Part model, mm, in its own coordinate system. Face numbers are marked on the shaded views. A direction names the side the tool comes from. Round coordinates to 2 decimals unless told otherwise and drop trailing zeros. Loops run counter-clockwise (first coordinate to the right, second up) from the corner with the lowest first, then second, coordinate; pieces in that order, holes last. Notation, with made-up numbers: M -2,32.5 L 37,32.5 A37 ccw 37,68.5 Z; hole C 55,28 d8. An arc over 180 degrees is marked long. Write each question's results on one line, items separated by ' | '.
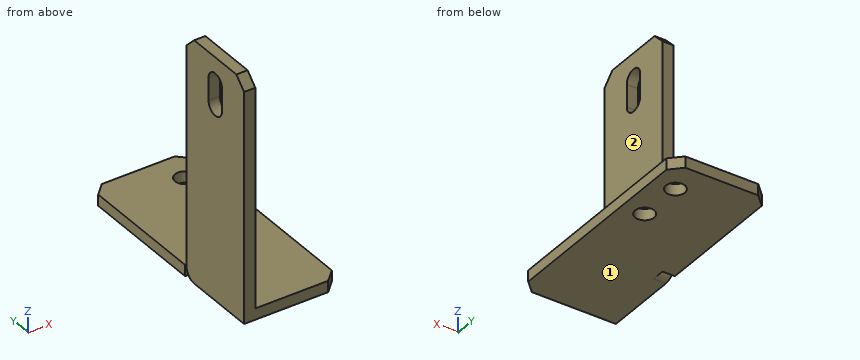
from build123d import *

# Parameters (mm, degrees)
SKETCH1_R           = 1.7
BOSS_EXTRUDE1_DEPTH = 2
SKETCH2_W           = 2
SKETCH2_H           = 15
BOSS_EXTRUDE2_DEPTH = 41
CUT_EXTRUDE1_DEPTH  = 52.818254684
FILLET1_R           = 2
CHAMFER1_SIZE       = 2


with BuildPart() as part:
    # Sketch1 → Boss-Extrude1 (new body)
    with BuildSketch(Plane.XY):
        Polygon((-8.078512397, -9.72107438), (-8.078512397, -24.72107438), (8.921487603, -24.72107438), (8.921487603, 15.27892562), (-8.078512397, 15.27892562), (-8.078512397, -9.36189554), (-5.878512397, -9.36189554), (-5.878512397, -9.72107438), align=None)
        with Locations((4.921487603, 9.77892562)):
            Circle(SKETCH1_R, mode=Mode.SUBTRACT)
        with Locations((4.921487603, 1.77892562)):
            Circle(SKETCH1_R, mode=Mode.SUBTRACT)
    extrude(amount=BOSS_EXTRUDE1_DEPTH)

    # Sketch2 → Boss-Extrude2 (add)
    with BuildSketch(Plane.XY.offset(2)):
        with Locations((-7.078512397, -17.22107438)):
            Rectangle(SKETCH2_W, SKETCH2_H)
    extrude(amount=BOSS_EXTRUDE2_DEPTH)

    # Sketch3 → Cut-Extrude1 (cut, through all)
    with BuildSketch(Plane(origin=(-6.078512397, 0, 0), x_dir=(0, 0, -1), z_dir=(1, 0, 0))):
        with BuildLine():
            Line((-38.423728751, -15.47107438), (-34.423728751, -15.47107438))
            ThreePointArc((-34.423728751, -15.47107438), (-32.673728751, -17.22107438), (-34.423728751, -18.97107438))
            Line((-34.423728751, -18.97107438), (-38.423728751, -18.97107438))
            ThreePointArc((-38.423728751, -18.97107438), (-40.173728751, -17.22107438), (-38.423728751, -15.47107438))
        make_face()
    extrude(amount=-CUT_EXTRUDE1_DEPTH, mode=Mode.SUBTRACT)

    # Fillet1
    fillet1_edges = [part.edges().sort_by_distance(p)[0] for p in [
        (-6.978512397, -9.72107438, 0),
    ]]
    fillet(fillet1_edges, radius=FILLET1_R - 0.0001)  # a hair under: the kernel refuses the full size

    # Chamfer1
    chamfer1_edges = [part.edges().sort_by_distance(p)[0] for p in [
        (-8.078512397, 15.27892562, 1),
        (8.921487603, 15.27892562, 1),
        (8.921487603, -24.72107438, 1),
        (-7.078512397, -24.72107438, 43),
        (-7.078512397, -9.72107438, 43),
    ]]
    chamfer(chamfer1_edges, length=CHAMFER1_SIZE)


solid = part.part
Item 1: Band-saw the part on B-B on x = 4.75. Give the cut face in (y, z), and give its area (3 significant figures).
Filled sheet:
outline: M -24.72,0 L 0.09,0 L 0.09,2 L -24.72,2 Z; M 3.47,0 L 8.09,0 L 8.09,2 L 3.47,2 Z; M 11.47,0 L 15.28,0 L 15.28,2 L 11.47,2 Z | area: 66.5 mm^2
Item 2: Band-saw the part on C-C on y = -4.5. Give the cut face in (x, z).
Filled sheet:
outline: M -8.08,0 L 8.92,0 L 8.92,2 L -8.08,2 Z
Item 3: Band-saw the part on D-D on z = 16.5. Give the cut face in (x, y), and give its area (3 significant figures).
Filled sheet:
outline: M -8.08,-24.72 L -6.08,-24.72 L -6.08,-9.72 L -8.08,-9.72 Z | area: 30.0 mm^2
Item 4: Wall check: L1, parallel to Y at x = -7, z = 37; L2, parallel to X at y = -12, z = 29; L3, parallel to Z at x = -2.25, y = -20. Give the ranges that are in metal, low to high.
Filled sheet:
L1: -24.72 to -18.97, -15.47 to -9.72 | L2: -8.08 to -6.08 | L3: 0 to 2
Item 5: Which spindle directions (+Z, -Z, +X, -X, +Y, -Y) get a long thin tool onto all of the face, cutting with end or side? Do the marked faces 1 and 2. Say none if no direction does.
Filled sheet:
face 1: -Z, +X, -X, +Y, -Y | face 2: +Z, +X, +Y, -Y
Item 6: Drop flat-ended pins along their axis: P1, Ø4, axis at x = 6, y = 1.5, coming from the +Z side; P2, Ø0.6, axis at x = -7.5, z = 36.5, coming from the +Y side; P3, Ø12, axis at y = -15, z = 21, coming from the +X side; P4, Ø5, axis at x = -1.5, z = 16, coming from the +Y side. Give the stop position or say it passes through.
Filled sheet:
P1: z = 2 | P2: y = -9.72 | P3: x = -6.08 | P4: through
Item 7: Band-saw the part on A-A on z = 37.5. Give the cut face in (x, y), and give its area (3 significant figures).
Filled sheet:
outline: M -8.08,-24.72 L -6.08,-24.72 L -6.08,-18.97 L -8.08,-18.97 Z; M -8.08,-15.47 L -6.08,-15.47 L -6.08,-9.72 L -8.08,-9.72 Z | area: 23.0 mm^2
